Source: CAD feature listing. Evaluate the final solid. Frame: model axes, mm. A direction names the side the tool comes from. Give positions to 0.01 mm unless a question says otherwise; leave off trailing zeros. Loops run counter-clockwise (first coordinate to the right, second up) from the corner with the lowest first, then second, coordinate; pieces in that order, holes last. Notation, with made-up numbers: M 17,83 L 35,83 A25 ccw 35,98 Z; hole C 0.5,40 d8. An arc over 180 degrees is marked long. Answer in a Markdown table with one row per item.
```python
from build123d import *

# Parameters (mm, degrees)
BASPROSKE_W        = 4.2
BASPROSKE_H        = 9.45
TOOTHCUT_DEPTH     = 15.008747267
TEETHCUTS_COUNT    = 25
TEETHCUTS_ANGLE    = 345.6
SKETCH7_R          = 2.4
CUT_EXTRUDE2_DEPTH = 1.6
SKETCH13_R         = 6.5
SKETCH13_R_2       = 3
CUT_EXTRUDE3_DEPTH = 1.2
CUT_EXTRUDE4_START = -1.2
SKETCH15_R         = 6.5
SKETCH15_R_2       = 3
CUT_EXTRUDE4_DEPTH = 1.2
CUT_EXTRUDE5_START = -1.6
SKETCH17_R         = 2.4
CUT_EXTRUDE5_DEPTH = 1.6
SKETCH18_R         = 0.9
CUT_EXTRUDE6_DEPTH = 1.6


with BuildPart() as part:
    # BasProSke → Base-Revolve (revolve)
    with BuildSketch(Plane(origin=(0, 0, 0), x_dir=(1, 0, 0), z_dir=(0, 1, 0)), mode=Mode.PRIVATE) as base_revolve_sk:
        with Locations((2.1, 4.725)):
            Rectangle(BASPROSKE_W, BASPROSKE_H)
    revolve(base_revolve_sk.sketch.rotate(Axis((-10, 0, 0), (1, 0, 0)), 180), axis=Axis((-10, 0, 0), (1, 0, 0)))

    # TooCutSke → ToothCut (cut, through all)
    with BuildSketch(Plane(origin=(0, 0, 0), x_dir=(0, 0, -1), z_dir=(1, 0, 0))):
        with BuildLine():
            ThreePointArc((0.336642775, 7.866800343), (0, 7.874), (-0.336642775, 7.866800343))
            ThreePointArc((-0.336642775, 7.866800343), (-0.577188207, 8.685445672), (-1.008672355, 9.421559597))
            ThreePointArc((-1.008672355, 9.421559597), (0, 9.4754), (1.008672355, 9.421559597))
            ThreePointArc((1.008672355, 9.421559597), (0.577188207, 8.685445672), (0.336642775, 7.866800343))
        make_face()
    toothcut = extrude(amount=TOOTHCUT_DEPTH, mode=Mode.SUBTRACT)

    # TeethCuts: ToothCut ×25 about axis
    teethcuts_axis = Axis((-10, 0, 0), (1, 0, 0))
    for i in range(1, TEETHCUTS_COUNT):
        add(toothcut.rotate(teethcuts_axis, i * TEETHCUTS_ANGLE / (TEETHCUTS_COUNT - 1)), mode=Mode.SUBTRACT)

    # Sketch7 → Cut-Extrude2 (cut)
    with BuildSketch(Plane(origin=(4.2, 0, 0), x_dir=(0, 0, -1), z_dir=(1, 0, 0))):
        Circle(SKETCH7_R)
    extrude(amount=-CUT_EXTRUDE2_DEPTH, mode=Mode.SUBTRACT)

    # Sketch13 → Cut-Extrude3 (cut)
    with BuildSketch(Plane(origin=(4.2, 0, 0), x_dir=(0, 0, -1), z_dir=(1, 0, 0))):
        Circle(SKETCH13_R)
        Circle(SKETCH13_R_2, mode=Mode.SUBTRACT)
    extrude(amount=-CUT_EXTRUDE3_DEPTH, mode=Mode.SUBTRACT)

    # Sketch15 → Cut-Extrude4 (cut)
    with BuildSketch(Plane.ZY.offset(CUT_EXTRUDE4_START)):
        with Locations(Location((0, 0, 0), (0, 0, 180))):
            Circle(SKETCH15_R)
        with Locations(Location((0, 0, 0), (0, 0, 180))):
            Circle(SKETCH15_R_2, mode=Mode.SUBTRACT)
    extrude(amount=CUT_EXTRUDE4_DEPTH, mode=Mode.SUBTRACT)

    # Sketch17 → Cut-Extrude5 (cut)
    with BuildSketch(Plane.ZY.offset(CUT_EXTRUDE5_START)):
        with Locations(Location((0, 0, 0), (0, 0, 180))):
            Circle(SKETCH17_R)
    extrude(amount=CUT_EXTRUDE5_DEPTH, mode=Mode.SUBTRACT)

    # Sketch18 → Cut-Extrude6 (cut)
    with BuildSketch(Plane(origin=(2.6, 0, 0), x_dir=(0, 0, -1), z_dir=(1, 0, 0))):
        Circle(SKETCH18_R)
    extrude(amount=-CUT_EXTRUDE6_DEPTH, mode=Mode.SUBTRACT)


solid = part.part
```
Q1. Contact query for flat-ended pins moving along their axis: pin 1 Ø7.5 at (y, z) = (0, 0) entering from +X; pin 2 Ø2 at (x, z) = (0.5, 5.5) entering from +Y; pin 3 Ø1 at (x, y) = (4, 3) entering from +Z; pin 4 Ø1 at (x, y) = (3.5, 7) entering from -Z. Output: stop coordinate, or through.
Values follow:
| item | result |
|---|---|
| pin 1 | x = 4.2 |
| pin 2 | y = 7.76 |
| pin 3 | z = 8.35 |
| pin 4 | z = -5.71 |
Q2. Reachability of faces 1 (the cylindrical face through (2.07, 8.27, -2.72)), 2 (the cylindrical face through (2.07, -7.86, 3.73)), 3 (the cylindrical face through (4, 0, 3)), 4 (the cylindrical face through (2.071, 8.53, -1.605)), 5 (the cylindrical face through (0.608, 3.955, 5.158)) from +Z, -Z, +X, -X, +Y, -Y: full face, straight path, thin tool, end or side. Return the list, or none.
Values follow:
| item | result |
|---|---|
| face 1 | +X, -X, +Y |
| face 2 | +X, -X, -Y |
| face 3 | +X |
| face 4 | +X, -X |
| face 5 | -X |
Q3. Mould query, pull axis Y, two halves, no side actions, for faces 6 (the cylindrical face through (2.071, 8.248, 2.703)), 7 (the cylindrical face through (2.071, -8.522, -1.648)), 8 (the flat face through (1.2, 1, -3)). Classes: +Y half, -Y half, draft (parallel to the pull), parting line (faces both ways), or undercut.
Values follow:
| item | result |
|---|---|
| face 6 | +Y half |
| face 7 | -Y half |
| face 8 | undercut |
Q4. Section query B-B (y = 3.25). Output: boundary loops of the cut face in (x, z), plus the area to 3 significant figures.
Values follow:
| item | result |
|---|---|
| outline | M 0,-8.1 L 4.2,-8.1 L 4.2,-5.63 L 3,-5.63 L 3,5.63 L 4.2,5.63 L 4.2,8.1 L 0,8.1 L 0,5.63 L 1.2,5.63 L 1.2,-5.63 L 0,-5.63 Z |
| area | 41.0 mm^2 |
Q5. Section query C-C (y = -5.5). Output: boundary loops of the cut face in (x, z).
Values follow:
| item | result |
|---|---|
| outline | M 0,-6.03 L 4.2,-6.03 L 4.2,-3.46 L 3,-3.46 L 3,3.46 L 4.2,3.46 L 4.2,6.03 L 0,6.03 L 0,3.46 L 1.2,3.46 L 1.2,-3.46 L 0,-3.46 Z |
Q6. Ray query, probe 1 along Y at (x, z) = (0.8, 0); probe 2 along Y at (x, z) = (0.2, 8.25); probe 3 along Z at (x, y) = (2.45, -8). Return the intervals inside material, ascending. Write a range as from..to.
Values follow:
| item | result |
|---|---|
| probe 1 | -9.45..-6.5, -3..-2.4, 2.4..3, 6.5..7.87 |
| probe 2 | -3.18..-2.08, -1.12..0.1, 0.95..2.15, 3.39..4.21 |
| probe 3 | -4.72..-3.88, -2.66..-1.4, -0.64..0.64, 1.4..2.66, 3.88..4.72 |
Q7. Section query A-A (x = 3.3). Give the number of separate pieces and of enclosed holes in the cut face, plus the area to 3 significant figures.
Values follow:
| item | result |
|---|---|
| separate pieces | 2 |
| enclosed holes | 2 |
| area | 111 mm^2 |
